Could you check a few things on this drawing? It's one solid part, dimensions in mm from its lowest x, y, z. A direction names the side the tool comes from. Round coordinates to 2 decimals unless told otherwise and drop trailing zeros. Write each loop counter-clockwise with the first axis right and the second up, starting at its lowest first coordinate (ties: lowest second). Pieces come first, ordered by that corner, then holes. Notation, with made-up numbers: (-28.75, 65.25) - (-11.75, 65.25) arc R16 ccw to (-11.75, 89.25) - close; hole circle Ø11 at (43, 62). An arc over 180 degrees is marked (long way). Put each result on its own line as item: value.
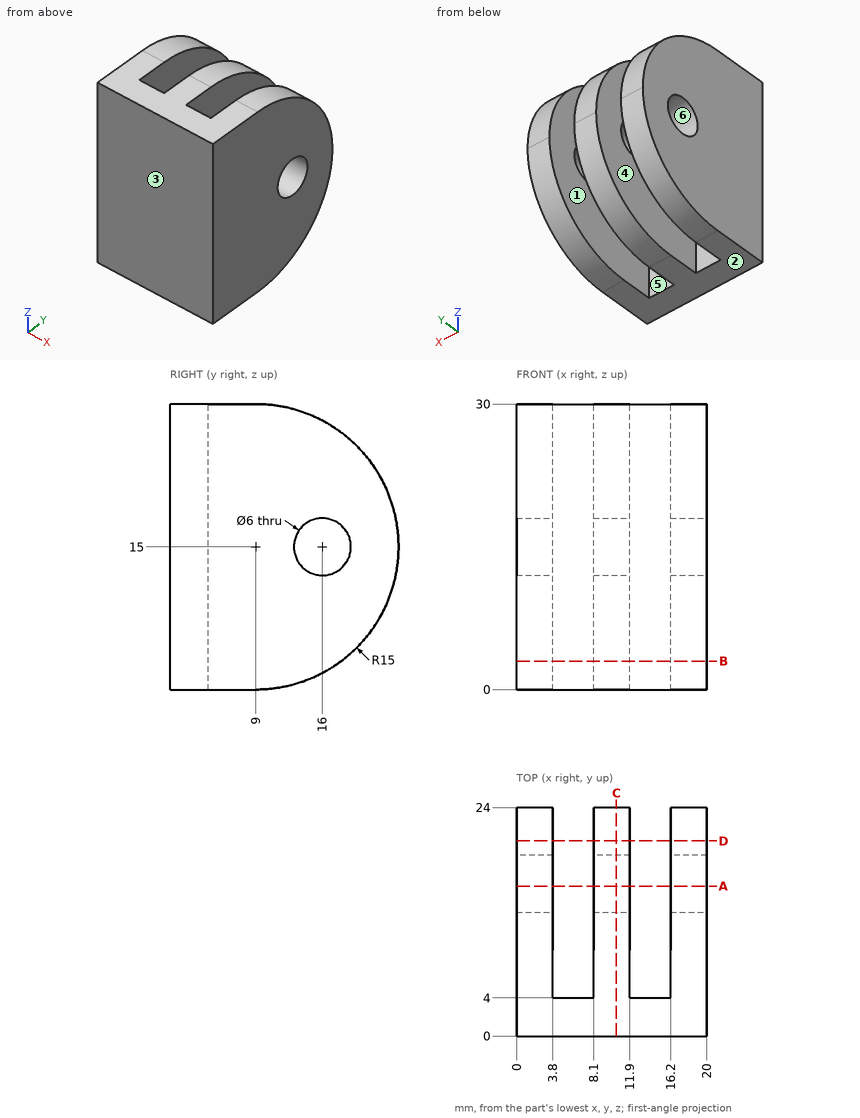
(1) Please list where these lines run through material, in increasing order: probe 1 along X at (y, z) = (11, 23); probe 2 along Y at (x, z) = (14.25, 4); probe 3 along Z at (x, y) = (2, 21). Write a range as from..to.
Values found:
probe 1: x = 0..3.8, 8.1..11.9, 16.2..20
probe 2: y = 0..4
probe 3: z = 6..24
(2) For the marked faces 1 and 2, which set-ups out of +Z, -Z, +X, -X, +Y, -Y let a thin tool reach every point of the face, with its end or its side?
Values found:
face 1: +Z, -Z, +Y
face 2: -Z, +X, -X, +Y, -Y
(3) If we mould it in two halves opening along Y, with no side actions, what happens to the marked faces 3, 4, 5 and 6? For each: pulls with the +Y half, pulls with the -Y half, needs draft (parallel to the pull), parting line crosses it, or undercut.
Values found:
face 3: pulls with the -Y half
face 4: needs draft
face 5: pulls with the +Y half
face 6: undercut
(4) Imagine slicing it at C-C, the plane x = 10.5. List the corners of the cut face in (y, z) for me.
Values found:
outline: (0, 0) - (9, 0) arc R15 ccw to (24, 15) arc R15 ccw to (9, 30) - (0, 30) - close; hole circle Ø6 at (16, 15)
(5) Imagine slicing it at A-A, the plane y = 15.75. List the corners of the cut face in (x, z) for me, then the cut area to 3 significant figures.
Values found:
outline: (0, 1.6) - (3.8, 1.6) - (3.8, 12.01) - (0, 12.01) - close; (0, 17.99) - (3.8, 17.99) - (3.8, 28.4) - (0, 28.4) - close; (8.1, 1.6) - (11.9, 1.6) - (11.9, 12.01) - (8.1, 12.01) - close; (8.1, 17.99) - (11.9, 17.99) - (11.9, 28.4) - (8.1, 28.4) - close; (16.2, 1.6) - (20, 1.6) - (20, 12.01) - (16.2, 12.01) - close; (16.2, 17.99) - (20, 17.99) - (20, 28.4) - (16.2, 28.4) - close
area: 237 mm^2
(6) Imagine slicing it at D-D, the plane y = 20.5. List the corners of the cut face in (x, z) for me, then the cut area to 3 significant figures.
Values found:
outline: (0, 5.37) - (3.8, 5.37) - (3.8, 24.63) - (0, 24.63) - close; (8.1, 5.37) - (11.9, 5.37) - (11.9, 24.63) - (8.1, 24.63) - close; (16.2, 5.37) - (20, 5.37) - (20, 24.63) - (16.2, 24.63) - close
area: 220 mm^2
(7) I'm going to push flat-ended pins straight in: pin 1 (4.5 mm diameter, centred on x = 6.5, z = 18.5, fed in from +Y); pin 2 (4.5 mm diameter, centred on x = 13.5, z = 17, fed in from +Y). Where does each tip first touch, or does it pass through?
Values found:
pin 1: stops at y = 23.88
pin 2: stops at y = 23.99
(8) Imagine slicing it at B-B, the plane z = 3. List the corners of the cut face in (x, y) for me.
Values found:
outline: (0, 0) - (20, 0) - (20, 18) - (16.2, 18) - (16.2, 4) - (11.9, 4) - (11.9, 18) - (8.1, 18) - (8.1, 4) - (3.8, 4) - (3.8, 18) - (0, 18) - close
